The model under review builds one solid part; all positions refer to its coordinate system, in mm. A direction names the side the tool comes from. Round coordinates to 2 decimals unless told otherwise and drop trailing zeros. Write each loop counter-clockwise with the first axis right and the second up, starting at its lowest first coordinate (ties: lowest second). Pieces come first, ordered by that corner, then holes. Notation, with made-up numbers: M 20,-15 L 49,-15 A24 cw 49,8 Z; hole C -2,76.5 d8. An arc over 180 degrees is marked long. One line per item, written item: value. Start each with the question number.
1) Wall thickness on probe 1 along Y at (x, z) = (-2.05, -12.7); probe 2 along Y at (x, z) = (-25.4, -1.7); probe 3 along Z at (x, y) = (-15, 23.5) (3 decimals): over which ranges is each line inside the solid? List them lowest first.
2) Take a section at D-D, the plane y = 62. Write out the cut boundary in (x, z) (3 decimals).
3) Mouldability with a two-part tool opening along Y and no side actions: class faces 4 (the face through (-1.57, 7.07, -14.97)), 5 (the face through (-3.175, 45, -13)), 6 (the face through (-25, 0, -2)), 7 (the face through (-25, 88.9, -2)) as +Y half, -Y half, draft (parallel to the pull), parting line (faces both ways), or undercut.
4) For P1, Ø23, axis at x = -25.4, y = 44.45, coming from the +Z side (3 decimals), flat-tipped, find the tip position at first contact; note if it passes through.
5) Take a section at C-C, the plane x = -25.4. Write out the cut boundary in (y, z) (1 decimal), and give its area (3 significant figures).
6) Take a section at B-B, the plane y = 6.35. Write out the cut boundary in (x, z) (3 decimals).
7) Take a section at A-A, the plane z = -12.7. Write out the cut boundary in (x, y) (3 decimals), and give its area (3 significant figures).
8) Tool access review of faces 1 (the face through (-1.57, 84.56, -13.98)), 2 (the face through (-47.625, 45, -13)), 3 (the face through (-35.93, 54.106, -1.565)): name each direction out of +Z, -Z, +X, -X, +Y, -Y from which nothing blocks a thin tool from reaching the whole face with its end or side.
Autodesk Inventor part; units mm, degrees
ref_plane "YZ Plane" through (0, 0, 0) normal (1, 0, 0) x (0, 1, 0)
ref_plane "XZ Plane" through (0, 0, 0) normal (0, 1, 0) x (-1, 0, 0)
ref_plane "XY Plane" through (0, 0, 0) normal (0, 0, 1) x (1, 0, 0)
sketch "Sketch3" plane through (0, 0, 0) normal (0, 1, 0) x (-1, 0, 0)
  line L0 (0, 0) -> (50.8, 0)
  line L1 (50.8, 0) -> (50.8, -25.4)
  line L2 (50.8, -25.4) -> (0, -25.4)
  line L3 (0, 0) -> (0, -25.4)
  dimension "d9" = 50.8
  dimension "d10" = 25.4
  dimension "d11" = 50.8
extrude "Extrusion3" add sketch "Sketch3" along normal blind 88.9
sketch "Sketch4" plane through (0, 88.9, 0) normal (0, 1, 0) x (1, 0, 0)
  line L0 (0, 25.4) -> (-50.8, 25.4)
  line L1 (-50.8, 25.4) -> (-50.8, 0)
  line L2 (-50.8, 0) -> (0, 0)
  line L3 (0, 0) -> (0, 25.4)
  line L4 (-47.625, 22.225) -> (-3.175, 22.225)
  line L5 (-3.175, 22.225) -> (-3.175, 3.175)
  line L6 (-3.175, 3.175) -> (-47.625, 3.175)
  line L7 (-47.625, 3.175) -> (-47.625, 22.225)
  dimension "d14" = 3.175
extrude "Extrusion4" cut sketch "Sketch4" against normal blind 88.9 contours L4 L5 L6 L7
sketch "Sketch5" plane through (-50.8, 0, 0) normal (0, 0, 1) x (1, 0, 0)
  line L0 (0, 0) -> (0, 88.9)
  line L1 (0, 0) -> (25.4, 0)
  line L2 (0, 0) -> (50.8, 0)
  line L3 (25.4, 0) -> (25.4, 44.45)
  circle A0 centre (25.4, 44.45) radius 14.2875
  dimension "d17" = 25.4
  dimension "d18" = 44.45
  dimension "d19" = 28.575
extrude "Extrusion5" cut sketch "Sketch5" against normal blind 3.175
sketch "Sketch6" plane through (0, 0, 0) normal (1, 0, 0) x (0, 0, -1)
  line L0 (0, 0) -> (25.4, 0)
  line L1 (0, 0) -> (12.7, 0)
  line L2 (12.7, 0) -> (12.7, 6.35)
  circle A0 centre (12.7, 6.35) radius 2.3813
  line L3 (25.4, 0) -> (25.4, 88.9)
  line L4 (12.7, 6.35) -> (12.7, 82.55)
  circle A1 centre (12.7, 82.55) radius 2.3813
  dimension "d22" = 12.7
  dimension "d23" = 6.35
  dimension "d24" = 4.7625
  dimension "d26" = 76.2
  dimension "d27" = 4.7625
extrude "Extrusion6" cut sketch "Sketch6" against normal up to surface (50.8 mm away)
properties part number "Bar"
Checked values:
1. probe 1: y = 0 to 3.97, 8.73 to 80.17, 84.93 to 88.9
1. probe 2: y = 0 to 30.16, 58.74 to 88.9
1. probe 3: z = -25.4 to -22.225, -3.175 to 0
2. outline: M -50.8,-25.4 L 0,-25.4 L 0,0 L -50.8,0 Z; hole M -47.625,-22.225 L -3.175,-22.225 L -3.175,-3.175 L -47.625,-3.175 Z
3. face 4: undercut
3. face 5: draft
3. face 6: -Y half
3. face 7: +Y half
4. P1: stops at z = -22.225
5. outline: M 0,-25.4 L 88.9,-25.4 L 88.9,-22.2 L 0,-22.2 Z; M 0,-3.2 L 30.2,-3.2 L 30.2,0 L 0,0 Z; M 58.7,-3.2 L 88.9,-3.2 L 88.9,0 L 58.7,0 Z
5. area: 474 mm2
6. outline: M -50.8,-25.4 L 0,-25.4 L 0,-15.081 L -3.175,-15.081 L -3.175,-22.225 L -47.625,-22.225 L -47.625,-15.081 L -50.8,-15.081 Z; M -50.8,-10.319 L -47.625,-10.319 L -47.625,-3.175 L -3.175,-3.175 L -3.175,-10.319 L 0,-10.319 L 0,0 L -50.8,0 Z
7. outline: M -50.8,0 L -47.625,0 L -47.625,3.969 L -50.8,3.969 Z; M -50.8,8.731 L -47.625,8.731 L -47.625,80.169 L -50.8,80.169 Z; M -50.8,84.931 L -47.625,84.931 L -47.625,88.9 L -50.8,88.9 Z; M -3.175,0 L 0,0 L 0,3.969 L -3.175,3.969 Z; M -3.175,8.731 L 0,8.731 L 0,80.169 L -3.175,80.169 Z; M -3.175,84.931 L 0,84.931 L 0,88.9 L -3.175,88.9 Z
7. area: 504 mm2
8. face 1: +X, -X
8. face 2: +Y, -Y
8. face 3: +Z
